Geometry: final body of the model. Coordinates: model frame, mm. A direction names the side the tool comes from. Coordinates: 2 decimals unless noted, no trailing zeros. Order: outer loops, then holes, each group sorted by start corner. A loop starts at its lowest first (then second) coordinate and runs counter-clockwise, first axis right, second up. Notation, with made-up numbers: (59, 68) -> (85, 68) arc R17 ccw to (85, 76) -> close; hole circle Ø7 at (30, 85.5). An arc over 180 degrees is marked (long way). Use one line per item in the form item = value.
```python
from build123d import *

# Parameters (mm, degrees)
F1_DEPTH    = 6
F2_T1_DEPTH = 10.3301270189
F2_T3_DEPTH = 11


# Not quite as in the source:
# - a fillet or chamfer that OpenCascade refuses, or shapes differently, is made with other operations: its cross-section is extruded or revolved along the edge and cut away or added


with BuildPart() as f1:
    # F0 (on Top) → F1 (new body)
    with BuildSketch(Plane.XY):
        Polygon((15, 0), (0, 0), (0, -4), (0, -6), (0.6717378856, -6), (15, -6), align=None)
        Polygon((0.6717378856, -6), (0, -6), (-0.5, -6), (-0.5, -14), (0, -14), (0.6717378856, -14), align=None)
        Polygon((15, -14), (0.6717378856, -14), (0, -14), (0, -16), (0, -20), (15, -20), align=None)
    extrude(amount=F1_DEPTH)

    # F2: fillet of radius 1 on 4 edges, made by hand

    # F2_s2 → F2_t1 (cut)
    with BuildSketch(Plane.XY.offset(-2.1650635095)):
        with BuildLine():
            ThreePointArc((0, -6), (-0.3660254038, -6.3660254038), (-0.5, -6.8660254038))
            Line((-0.5, -6.8660254038), (-0.5, -6))
            Line((-0.5, -6), (0, -6))
        make_face()
        with BuildLine():
            ThreePointArc((-0.5, -13.1339745962), (-0.3660254038, -13.6339745962), (0, -14))
            Line((0, -14), (-0.5, -14))
            Line((-0.5, -14), (-0.5, -13.1339745962))
        make_face()
    extrude(amount=F2_T1_DEPTH, mode=Mode.SUBTRACT)

    # F2_s4 → F2_t3 (cut)
    with BuildSketch(Plane.XY.offset(-2.5)):
        with BuildLine():
            ThreePointArc((1, 0), (0.2928932188, -0.2928932188), (0, -1))
            Line((0, -1), (0, 0))
            Line((0, 0), (1, 0))
        make_face()
        with BuildLine():
            ThreePointArc((0, -19), (0.2928932188, -19.7071067812), (1, -20))
            Line((1, -20), (0, -20))
            Line((0, -20), (0, -19))
        make_face()
    extrude(amount=F2_T3_DEPTH, mode=Mode.SUBTRACT)


solid = f1.part
```
1) Section B-B, the plane z = 2.3. Output: boundary loops of the cut face in (x, y).
Results found:
outline = (-0.5, -13.13) arc R1 ccw to (0, -14) -> (0, -19) arc R1 ccw to (1, -20) -> (15, -20) -> (15, -14) -> (0.67, -14) -> (0.67, -6) -> (15, -6) -> (15, 0) -> (1, 0) arc R1 ccw to (0, -1) -> (0, -6) arc R1 ccw to (-0.5, -6.87) -> close
2) Section C-C, the plane y = -3.25. Output: boundary loops of the cut face in (x, z).
Results found:
outline = (0, 0) -> (15, 0) -> (15, 6) -> (0, 6) -> close
3) Section A-A, the plane x = 11.25. Output: boundary loops of the cut face in (y, z), and give its area (3 significant figures).
Results found:
outline = (-20, 0) -> (-14, 0) -> (-14, 6) -> (-20, 6) -> close; (-6, 0) -> (0, 0) -> (0, 6) -> (-6, 6) -> close
area = 72.0 mm2
4) Access query for faces 1 (the flat face through (7, -5, 0)), 2 (the flat face through (-0.5, -10, 3)), 3 (the flat face through (0, -3, 3)), 4 (the flat face through (0, -16, 3)), 5 (the flat face through (8, -14, 3)). Directions: +Z, -Z, +X, -X, +Y, -Y. A direction counts if a zero-diameter tool reaches every point of the face in a straight line with its end or side. Return the directions, or none.
Results found:
face_1 = -Z, +X, -X, +Y, -Y
face_2 = +Z, -Z, -X, +Y, -Y
face_3 = +Z, -Z, -X, +Y
face_4 = +Z, -Z, -X, -Y
face_5 = +Z, -Z, +X
5) Material intervals for probe 1 along Y at (x, z) = (7.5, 3.45); probe 2 along X at (y, z) = (-15.5, 4.95); probe 3 along X at (y, z) = (-10, 0.35), sorted ascending. Write a range as from..to.
Results found:
probe_1 = -20..-14, -6..0
probe_2 = 0..15
probe_3 = -0.5..0.67
6) Pull-direction query (Y, two-part tool) for faces 6 (the flat face through (8, -6, 3)), 7 (the flat face through (15, -3, 3)), 8 (the flat face through (8, 0, 3)); classes: released by +Y, released by -Y, zero draft, split by the parting line, or undercut.
Results found:
face_6 = undercut
face_7 = zero draft
face_8 = released by +Y
7) Contact query for a flat-ended pin moving along its axis: P1, Ø3, axis at x = 10.5, z = 4, coming from the +Y side. Output: stop coordinate, or through.
Results found:
P1 = 0
8) Section D-D, the plane y = -13.5. Output: boundary loops of the cut face in (x, z).
Results found:
outline = (-0.43, 0) -> (0.67, 0) -> (0.67, 6) -> (-0.43, 6) -> close
